Check sheet for the modelled part. Datum: model origin and axes. Units: mm. Round coordinates to 2 decimals unless told otherwise and drop trailing zeros. Loops run counter-clockwise (first coordinate to the right, second up) from the corner with the lowest first, then second, coordinate; pieces in that order, holes last. Notation, with made-up numbers: (-37.5, 60.5) - (8.5, 60.5) arc R14 cw to (8.5, 71.5) - close; hole circle Ø5 at (84.25, 17.25). An arc over 180 degrees is marked (long way). Return JSON: item names as keys, results as strings.
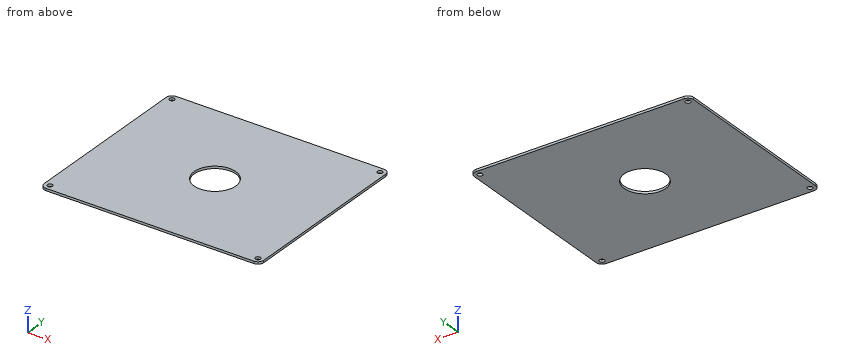
Autodesk Inventor part; units mm, degrees
ref_plane "YZ Plane" through (0, 0, 0) normal (1, 0, 0) x (0, 1, 0)
ref_plane "XZ Plane" through (0, 0, 0) normal (0, 1, 0) x (-1, 0, 0)
ref_plane "XY Plane" through (0, 0, 0) normal (0, 0, 1) x (1, 0, 0)
sketch "Sketch1" plane through (0, 0, 0) normal (0, 0, 1) x (1, 0, 0)
  line L0 (-45, -40) -> (45, -40)
  line L1 (47.5, -37.5) -> (47.5, 37.5)
  line L2 (45, 40) -> (-45, 40)
  line L3 (-47.5, 37.5) -> (-47.5, -37.5)
  line L4 (-47.5, -40) -> (47.5, 40) construction
  line L5 (47.5, -40) -> (-47.5, 40) construction
  arc A0 (-45, 40) -> (-47.5, 37.5) centre (-45, 37.5) ccw
  arc A1 (47.5, 37.5) -> (45, 40) centre (45, 37.5) ccw
  arc A2 (45, -40) -> (47.5, -37.5) centre (45, -37.5) ccw
  arc A3 (-47.5, -37.5) -> (-45, -40) centre (-45, -37.5) ccw
  point P0 (0, 0)
  dimension "d0" = 95
  dimension "d1" = 80
  dimension "d2" = 2.5
extrude "Extrusion1" add sketch "Sketch1" along normal mid plane 1
sketch "Sketch2" plane through (0, 0, -0.5) normal (0, 0, -1) x (-1, 0, 0)
  circle A0 centre (0, 0) radius 9
  dimension "d5" = 18
extrude "Extrusion2" cut sketch "Sketch2" against normal through all
sketch "Sketch3" plane through (0, 0, -0.5) normal (0, 0, -1) x (-1, 0, 0)
  circle A0 centre (0, 0) radius 9
  line L0 (47.5, -37.5) -> (47.5, 37.5)
  arc A1 (47.5, 37.5) -> (45, 40) centre (45, 37.5) ccw
  line L1 (45, 40) -> (-45, 40)
  arc A2 (-45, 40) -> (-47.5, 37.5) centre (-45, 37.5) ccw
  line L2 (-47.5, 37.5) -> (-47.5, -37.5)
  arc A3 (-47.5, -37.5) -> (-45, -40) centre (-45, -37.5) ccw
  line L3 (-45, -40) -> (45, -40)
  arc A4 (45, -40) -> (47.5, -37.5) centre (45, -37.5) ccw
hole "Hole1" at (-45, -37.5, -0.5) at (45, -37.5, -0.5) at (45, 37.5, -0.5) at (-45, 37.5, -0.5) direction (0, 0, 1) diameter 2.2 end through all
properties part number "Structure_-ZCover" material "Aluminum 6061"
Q1. Sectioned sample at B-B (x = 0). Enter the section's corners in (y, z), plus the area to 3 significant figures.
Answer key:
{"outline": "(-40, -0.5) - (-9, -0.5) - (-9, 0.5) - (-40, 0.5) - close; (9, -0.5) - (40, -0.5) - (40, 0.5) - (9, 0.5) - close", "area": "62.0 mm²"}
Q2. Sectioned sample at C-C (z = 0.3). Enter the section's corners in (x, y).
Answer key:
{"outline": "(-47.5, -37.5) arc R2.5 ccw to (-45, -40) - (45, -40) arc R2.5 ccw to (47.5, -37.5) - (47.5, 37.5) arc R2.5 ccw to (45, 40) - (-45, 40) arc R2.5 ccw to (-47.5, 37.5) - close; hole circle Ø2.2 at (-45, -37.5); hole circle Ø2.2 at (-45, 37.5); hole circle Ø18 at (0, 0); hole circle Ø2.2 at (45, -37.5); hole circle Ø2.2 at (45, 37.5)"}
Q3. Sectioned sample at A-A (y = 0). Enter the section's corners in (x, z).
Answer key:
{"outline": "(-47.5, -0.5) - (-9, -0.5) - (-9, 0.5) - (-47.5, 0.5) - close; (9, -0.5) - (47.5, -0.5) - (47.5, 0.5) - (9, 0.5) - close"}
Q4. Depth check by flat-ended pin: P1, Ø1.8, axis at x = -45, y = -37.5, coming from the -Z side. Enter the tip coordinate at first touch or a pass-through.
Answer key:
{"P1": "passes through"}
Q5. Scan lines: probe 1 along Y at (x, z) = (-45, -0.2); probe 2 along X at (y, z) = (37.5, 0.2); probe 3 along Y at (x, z) = (0, -0.05). Record each from-to range of solid material in increasing order. Write a range as [from, to].
Answer key:
{"probe 1": "y = [-40, -38.6], [-36.4, 36.4], [38.6, 40]", "probe 2": "x = [-47.5, -46.1], [-43.9, 43.9], [46.1, 47.5]", "probe 3": "y = [-40, -9], [9, 40]"}
